```python
from build123d import *

# Parameters (mm, degrees)
F0_W      = 62.0650928468
F0_H      = 90.1293121278
F1_DEPTH  = 42.672
F2_W      = 48.5726818442
F2_H      = 77.7162946761
F3_DEPTH  = 76.454
F4_W      = 48.5726818442
F4_H      = 77.7162946761
F5_DEPTH  = 0.762
F7_D      = 20.32
F8_W      = 52.8902541846
F8_H      = 23.0720248073
F9_DEPTH  = 43.688
F10_W     = 52.6204034686
F10_H     = 17.9449077696
F12_DEPTH = 25.4
F13_W     = 48.8425306976
F13_H     = 17.1353630722
F14_DEPTH = 25.4


with BuildPart() as f1:
    # F0 (on Top) → F1 (new body)
    with BuildSketch(Plane.XY):
        with Locations((2.9683308676, -0.9444709867)):
            Rectangle(F0_W, F0_H)
    extrude(amount=F1_DEPTH)

    # F2 (on Top) → F3 (cut)
    with BuildSketch(Plane.XY):
        with Locations((3.1032543629, -0.5396958441)):
            Rectangle(F2_W, F2_H)
    extrude(amount=F3_DEPTH, mode=Mode.SUBTRACT)

    # F4 (on face) → F5 (join)
    with BuildSketch(Plane.XY.offset(42.672)):
        with Locations((3.1032543629, -0.5396958441)):
            Rectangle(F4_W, F4_H)
    extrude(amount=-F5_DEPTH)

    # F7 (through all)
    with Locations(Plane.XZ.offset(46.0091270506)):
        with Locations((4.317572806, 18.754452467)):
            Hole(F7_D / 2)

    # F8 (on face) → F9 (cut)
    with BuildSketch(Plane.YZ.offset(34.000877291)):
        with Locations((-2.4286350235, 11.5360124037)):
            Rectangle(F8_W, F8_H)
    extrude(amount=F9_DEPTH, mode=Mode.SUBTRACT)

    # F10 (on face) → F12 (cut)
    with BuildSketch(Plane(origin=(-28.0642155558, 0, 0), x_dir=(0, -1, 0), z_dir=(-1, 0, 0))):
        with Locations((-0.134922564, 8.9724538848)):
            Rectangle(F10_W, F10_H)
    extrude(amount=-F12_DEPTH, mode=Mode.SUBTRACT)

    # F13 (on face) → F14 (cut)
    with BuildSketch(Plane.YZ.offset(34.000877291)):
        with Locations((0.1349244267, 8.5676815361)):
            Rectangle(F13_W, F13_H)
    extrude(amount=-F14_DEPTH, mode=Mode.SUBTRACT)


solid = f1.part
```
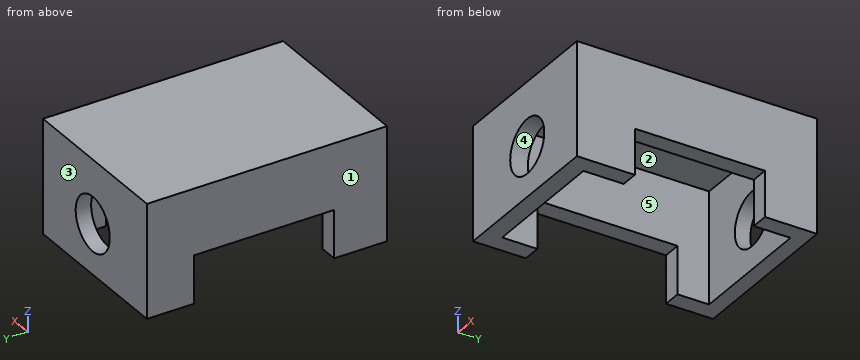
Geometry check sheet. Reference: the model listing, model coordinates, mm. Face numbers are marked on the shaded views. A direction names the side the tool comes from. Round coordinates to 2 decimals unless told otherwise and drop trailing zeros. Loops run counter-clockwise (first coordinate to the right, second up) from the corner with the lowest first, then second, coordinate; pieces in that order, holes last. Notation, with made-up numbers: (34, -38.5) - (74, -38.5) arc R24 ccw to (74, -1.5) - close; hole circle Ø3 at (0, -38.75). An arc over 180 degrees is marked (long way). Write item = value, one per line. Start each with the question number.
1. Section check D-D on x = 20. Enter the section's corners in (y, z).
2. Section check A-A on z = 31. Enter the section's corners in (x, y).
3. Set-up check for the marked faces 1 and 2: record each of +Z, -Z, +X, -X, +Y, -Y from which the full face is reachable in a straight line by a thin tool's end or side.
4. Section check B-B on x = 13.5. Enter the section's corners in (y, z), then the cut area to 3 significant figures.
5. Depth check by flat-ended pin: pin 1 (5 mm diameter, centred on x = 0.5, y = -29.5, fed in from -Z); pin 2 (2 mm diameter, centred on x = 31, y = -5.5, fed in from -Z); pin 3 (5.5 mm diameter, centred on x = -23.5, y = -3.5, fed in from -Z). Enter the tip coordinate at first touch or a pass-through.
6. Mould release check, pull along Y, two halves, no side actions. Record for the marked faces 3, 4 and 5: released by +Y, released by -Y, zero draft, split by the parting line, or undercut.
7. Section check C-C on y = -14.5. Enter the section's corners in (x, z), then the cut area to 3 significant figures.
8. Thickness scan on line 1 (Y direction, x = 22, z = 37); line 2 (X direction, y = -31, z = 3); line 3 (Y direction, x = -25, z = 7). Record the ranges inside material, lowest first.
Working result:
q1.outline = (-46.01, 0) - (-39.4, 0) - (-39.4, 41.91) - (38.32, 41.91) - (38.32, 0) - (44.12, 0) - (44.12, 42.67) - (-46.01, 42.67) - close
q2.outline = (-28.06, -46.01) - (34, -46.01) - (34, 44.12) - (-28.06, 44.12) - close; hole (-21.18, -39.4) - (27.39, -39.4) - (27.39, 38.32) - (-21.18, 38.32) - close
q3.face_1 = +Z, -Z, -X, +Y, -Y
q3.face_2 = -Z
q4.outline = (-46.01, 0) - (-39.4, 0) - (-39.4, 14.41) - (-46.01, 14.41) - close; (-46.01, 23.1) - (-39.4, 23.1) - (-39.4, 41.91) - (38.32, 41.91) - (38.32, 23.1) - (44.12, 23.1) - (44.12, 42.67) - (-46.01, 42.67) - close; (38.32, 0) - (44.12, 0) - (44.12, 14.41) - (38.32, 14.41) - close
q4.area = 481 mm^2
q5.pin_1 = 41.91
q5.pin_2 = 17.14
q5.pin_3 = 17.94
q6.face_3 = released by +Y
q6.face_4 = zero draft
q6.face_5 = undercut
q7.outline = (-28.06, 17.94) - (-21.18, 17.94) - (-21.18, 41.91) - (27.39, 41.91) - (27.39, 17.14) - (34, 17.14) - (34, 42.67) - (-28.06, 42.67) - close
q7.area = 376 mm^2
q8.line_1 = -46.01 to -39.4, 38.32 to 44.12
q8.line_2 = -28.06 to -21.18, 27.39 to 34
q8.line_3 = -46.01 to -26.18, 26.45 to 44.12
